Geometry check sheet. Reference: the model listing, model coordinates, mm. Coordinates: 2 decimals unless noted, no trailing zeros. Loops run counter-clockwise (first coordinate to the right, second up) from the corner with the lowest first, then second, coordinate; pieces in that order, holes last.
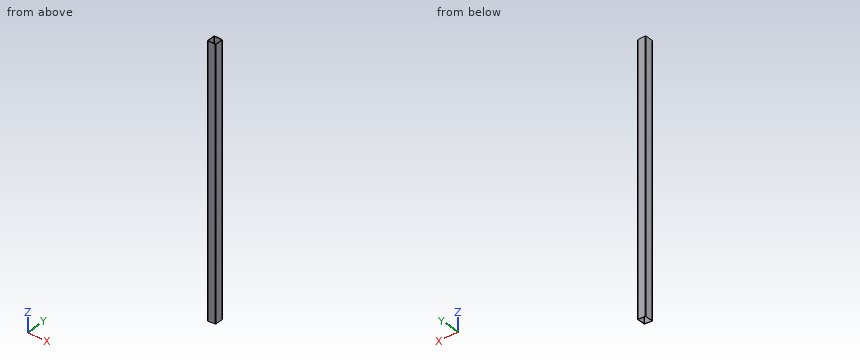
Autodesk Inventor part; units mm, degrees
ref_plane "Start Plane" through (0, 0, 160.6598) normal (0, 0, 1) x (1, 0, 0)
ref_plane "End Plane" through (0, 0, 2720) normal (0, 0, 1) x (1, 0, 0)
ref_plane "Work Plane4" through (2145.5143, 34, 359.3429) normal (0.0905357, 0, -0.9958932) x (-0.9958932, 0, -0.0905357)
ref_plane "Start Plane" through (0, 0, 160.6598) normal (0, 0, 1) x (1, 0, 0)
ref_plane "End Plane" through (0, 0, 2720) normal (0, 0, 1) x (1, 0, 0)
sketch "Sketch" plane through (0, 0, 0) normal (0, 0, 1) x (1, 0, 0)
  line L0 (-40, -34) -> (-40, 34)
  line L1 (-34, 40) -> (34, 40)
  line L2 (40, 34) -> (40, -34)
  line L3 (34, -40) -> (-34, -40)
  arc A0 (-40, -34) -> (-34, -40) centre (-34, -34) ccw
  arc A1 (40, 34) -> (34, 40) centre (34, 34) ccw
  arc A2 (-34, 40) -> (-40, 34) centre (-34, 34) ccw
  arc A3 (34, -40) -> (40, -34) centre (34, -34) ccw
  arc A4 (-34, 37) -> (-37, 34) centre (-34, 34) ccw
  line L4 (-34, 37) -> (34, 37)
  arc A5 (37, 34) -> (34, 37) centre (34, 34) ccw
  line L5 (37, 34) -> (37, -34)
  arc A6 (34, -37) -> (37, -34) centre (34, -34) ccw
  line L6 (34, -37) -> (-34, -37)
  arc A7 (-37, -34) -> (-34, -37) centre (-34, -34) ccw
  line L7 (-37, -34) -> (-37, 34)
  line L8 (0, 57.7397) -> (0, -57.7397) construction
  line L9 (-57.7397, 0) -> (57.7397, 0) construction
  dimension "d7" = 6
  dimension "d9" = 80
  dimension "d11" = 80
  dimension "d12" = 3
  dimension "d15" = 40
  dimension "d16" = 40
extrude "Body" add sketch "Sketch" along normal up to surface (2559.3402 mm away) from surface at 160.6598
sketch "Sketch3" plane through (0, 0, 0) normal (0, 0, 1) x (1, 0, 0)
  line L0 (0, 0) -> (10, 0)
ref_plane "Work Plane3" through (0, 0, 0) normal (0, -1, 0) x (1, 0, 0)
ref_plane "Work Plane4" through (2145.5143, 34, 359.3429) normal (0.0905357, 0, -0.9958932) x (-0.9958932, 0, -0.0905357)
split "Split1" plane through (2145.5143, 34, 359.3429) removes the side toward (0.0905357, 0, -0.9958932)
sketch "Sketch4" plane through (0, 0, 0) normal (0, -1, 0) x (1, 0, 0)
  line L0 (-2, 160.6598) -> (12, 160.6598)
  line L1 (-2, 2720) -> (12, 2720)
  dimension "d18" = 2559.3402
equation "\"d7\" = G_IR"
equation "\"d9\" = G_W"
equation "\"d11\" = G_H"
equation "\"d12\" = G_T"
equation "\"d15\" = 0.5 * d9"
equation "\"d16\" = 0.5 * d11"
equation "\"d3\" = G_L"
equation "\"G_W\" = 80"
equation "\"G_H\" = 80"
equation "\"G_T\" = 3"
equation "\"G_IR\" = 6"
equation "\"G_L\" = d18"
equation "\"G_OFFSET_START\" = -160.6598"
equation "\"d13\" = -G_OFFSET_START"
properties part number "ISO 10799-2 - 80x80x3 - 2559,34" material "Steel, Mild"
(1) Sectioned sample at C-C on z = 1309.5. Record the cut outline in (x, y).
Findings:
outline: (-40, -34) arc R6 ccw to (-34, -40) - (34, -40) arc R6 ccw to (40, -34) - (40, 34) arc R6 ccw to (34, 40) - (-34, 40) arc R6 ccw to (-40, 34) - close; hole (-37, -34) arc R3 ccw to (-34, -37) - (34, -37) arc R3 ccw to (37, -34) - (37, 34) arc R3 ccw to (34, 37) - (-34, 37) arc R3 ccw to (-37, 34) - close
(2) Sectioned sample at A-A on y = 19.5. Record the cut outline in (x, z), and give its area (3 significant figures).
Findings:
outline: (-40, 160.66) - (-37, 160.93) - (-37, 2720) - (-40, 2720) - close; (37, 167.66) - (40, 167.93) - (40, 2720) - (37, 2720) - close
area: 15,300 mm2
(3) Scan lines: L1, parallel to Y at x = 12.5, z = 653; L2, parallel to X at y = -36.5, z = 1007. Record each from-to range of solid material in increasing order.
Findings:
L1: y = -40 to -37, 37 to 40
L2: x = -39.45 to -35.66, 35.66 to 39.45
(4) Sectioned sample at B-B on x = -21. Record the cut outline in (y, z), and give its area (3 significant figures).
Findings:
outline: (-40, 162.39) - (-37, 162.39) - (-37, 2720) - (-40, 2720) - close; (37, 162.39) - (40, 162.39) - (40, 2720) - (37, 2720) - close
area: 15,300 mm2
